Autodesk Inventor part; units mm, degrees
ref_plane "YZ Plane" through (0, 0, 0) normal (1, 0, 0) x (0, 1, 0)
ref_plane "XZ Plane" through (0, 0, 0) normal (0, 1, 0) x (-1, 0, 0)
ref_plane "XY Plane" through (0, 0, 0) normal (0, 0, 1) x (1, 0, 0)
sketch "Esquisse1" plane through (0, 0, 0) normal (0, 1, 0) x (-1, 0, 0)
  circle A0 centre (0, 0) radius 31
  circle A1 centre (0, 0) radius 50
  circle A2 centre (0, 0) radius 40
  line L0 (45, -21.7945) -> (45, 21.7945)
  dimension "d0" = 62
  dimension "d1" = 100
  dimension "d2" = 80
  dimension "d47" = 45
extrude "Extrusion1" add sketch "Esquisse1" along normal blind 5 contours A1 L0 | L0 A1 | A2
sketch "Esquisse2" plane through (0, 5, 0) normal (0, 1, 0) x (1, 0, 0)
  circle A0 centre (0, 0) radius 40
  circle A1 centre (0, 0) radius 31
  circle A2 centre (0, 0) radius 31
  dimension "d6" = 80
  dimension "d75" = 0
extrude "Extrusion2" add sketch "Esquisse2" along normal blind 26.3
sketch "Esquisse3" plane through (0, 31.3, 0) normal (0, 1, 0) x (1, 0, 0)
  circle A0 centre (0, 0) radius 20
  circle A1 centre (0, 0) radius 40
  circle A2 centre (0, 0) radius 40
  dimension "d9" = 40
  dimension "d63" = 0
extrude "Extrusion3" add sketch "Esquisse3" along normal blind 5
sketch "Esquisse5" plane through (0, 36.3, 0) normal (0, 1, 0) x (1, 0, 0)
  line L0 (-33, 22.6053) -> (-33, -22.6053)
  circle A0 centre (0, 0) radius 40
  circle A1 centre (0, 0) radius 40
  point P0 (-33, 22.6053)
  dimension "d71" = 80
  dimension "d72" = 33
extrude "Extrusion4" cut sketch "Esquisse5" against normal up to surface (31.3 mm away) contours L0 A0 picked at (-34.2788, -5.1971)
sketch "Esquisse6" plane through (0, 5, 0) normal (0, 1, 0) x (1, 0, 0)
  point P0 (0, 0)
sketch "Esquisse7" plane through (0, 5, 0) normal (0, 1, 0) x (1, 0, 0)
  line L0 (12, 65.0926) -> (12, -68.5298) construction
  circle A0 centre (0, 0) radius 20 construction
  circle A1 centre (12, 43) radius 3.5
  circle A2 centre (12, -43) radius 3.5
  point P0 (-37.5, -12.5)
  point P1 (-37.5, 12.5)
  dimension "d53" = 12
  dimension "d54" = 7
  dimension "d55" = 7
  dimension "d56" = 43
  dimension "d57" = 43
extrude "Extrusion6" cut sketch "Esquisse7" against normal blind 10
sketch "Esquisse8" plane through (0, 5, 0) normal (0, 1, 0) x (1, 0, 0)
  line L0 (-45, 21.7945) -> (-45, -21.7945)
  circle A0 centre (0, 0) radius 50
  dimension "d73" = 45
  dimension "d74" = 100
extrude "Extrusion7" cut sketch "Esquisse8" against normal blind 5 contours L0 A0 picked at (-46.0601, 4.4554)
sketch "Esquisse9" plane through (0, 5, 0) normal (0, 1, 0) x (1, 0, 0)
  line L0 (41, 168.1574) -> (41, -90.4051) construction
  circle A0 centre (41, 18) radius 3.5
  circle A1 centre (41, -18) radius 3.5
  circle A2 centre (0, 0) radius 20
  dimension "d58" = 7
  dimension "d59" = 7
  dimension "d60" = 18
  dimension "d61" = 18
  dimension "d62" = 41
extrude "Extrusion8" cut sketch "Esquisse9" against normal blind 5 contours A0 | A1
sketch "Sketch10" plane through (0, 0, 0) normal (0, -1, 0) x (1, 0, 0)
  line L0 (-39, -54.8136) -> (-39, 70.7566) construction
  circle A0 centre (-39, -20) radius 3.5
  circle A1 centre (-39, 20) radius 3.5
  point P0 (0, 0)
  dimension "d64" = 39
  dimension "d65" = 20
  dimension "d66" = 20
  dimension "d67" = 7
  dimension "d68" = 7
extrude "Extrusion9" cut sketch "Sketch10" against normal blind 5
equation "\"d55\" = d54"
equation "\"d57\" = d56"
equation "\"d59\" = d58"
equation "\"d61\" = d60"
equation "\"d68\" = d67"
properties part number "B1 fixe2"
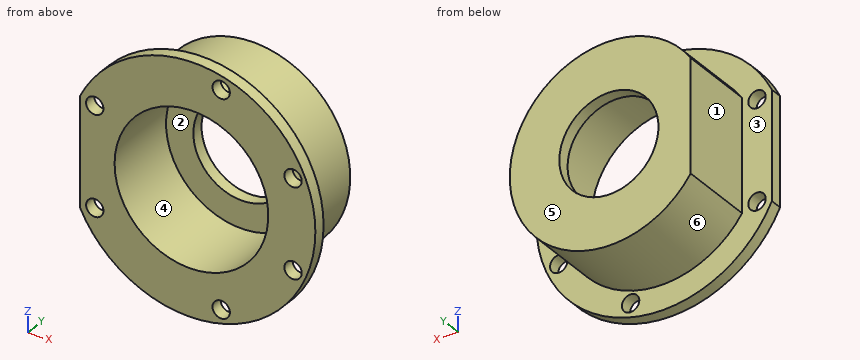
The model under review builds one solid part; all positions refer to its coordinate system, in mm. Face numbers are marked on the shaded views. A direction names the side the tool comes from. Give positions to 0.01 mm unless a question says otherwise; leave off trailing zeros. Loops run counter-clockwise (first coordinate to the right, second up) from the corner with the lowest first, then second, coordinate; pieces in that order, holes last. Notation, with made-up numbers: (-16, 85) -> (1, 85) arc R31 ccw to (1, 109) -> close; hole circle Ø1 at (29, -28). An arc over 180 degrees is marked (long way). Use CSV: the item, a comma, the result in double quotes.
1. The part is to be moulded in two halves that separate along X. For the marked faces 1, 2 and 3, say which applies: +X half, -X half, draft (parallel to the pull), parting line (faces both ways), or undercut.
Result:
face 1,"-X half"
face 2,"undercut"
face 3,"draft"
2. Consider section A-A, the plane z = -18. Write out the cut boundary in (x, y).
Result:
outline,"(-45, 0) -> (-41.87, 0) -> (-41.87, 5) -> (-45, 5) -> close; (-36.13, 0) -> (-25.24, 0) -> (-25.24, 31.3) -> (-8.72, 31.3) -> (-8.72, 36.3) -> (-33, 36.3) -> (-33, 5) -> (-36.13, 5) -> close; (8.72, 31.3) -> (25.24, 31.3) -> (25.24, 0) -> (37.5, 0) -> (37.5, 5) -> (35.72, 5) -> (35.72, 36.3) -> (8.72, 36.3) -> close; (44.5, 0) -> (46.65, 0) -> (46.65, 5) -> (44.5, 5) -> close"
3. Consider section C-C, the plane y = 20. Write out the cut boundary in (x, z), then the cut area to 3 significant figures.
Result:
outline,"(-33, -22.61) arc R40 ccw (long way) to (-33, 22.61) -> close; hole circle Ø62 at (0, 0)"
area,"1,790 mm²"
4. To check wall thickness, follow probe 1 along Z at (x, y) = (12, 2.8); probe 2 along Z at (x, y) = (41, 3.8); probe 3 along Z at (x, y) = (-39, 3.95). State the ranges of each line that lie inside material, in increasing order. Write a range as from..to.
Result:
probe 1,"z = -48.54..-46.5, -39.5..-28.58, 28.58..39.5, 46.5..48.54"
probe 2,"z = -28.62..-21.5, -14.5..14.5, 21.5..28.62"
probe 3,"z = -31.29..-23.5, -16.5..16.5, 23.5..31.29"
5. Machinability: for the marked faces 4, 5 and 6, which of the approach directions +Z, -Z, +X, -X, +Y, -Y give a long, thin tool a straight path to every point of the face, cutting with its end or side? Answer none if there is none.
Result:
face 4,"-Y"
face 5,"+Z, -Z, +X, -X, +Y"
face 6,"+Y"
6. For P1, Ø2, axis at y = 6.5, z = -21, coming from the +X side; P2, Ø1.5, axis at x = 5, y = 21.5, coming from the +Z side; P3, Ø2, axis at x = 14, y = 29.5, coming from the -Z side, all flat-tipped, find the tip position at first contact; note any pin that passes through.
Result:
P1,"stops at x = 34.64"
P2,"stops at z = 39.77"
P3,"stops at z = -37.83"
